Could you check a few things on this model? Use its own coordinates, in mm. Give positions to 0.01 mm unless a question says otherwise; leave off trailing zeros. Loops run counter-clockwise (first coordinate to the right, second up) from the corner with the lowest first, then second, coordinate; pieces in that order, holes last.
1. Imagine slicing it at D-D (y = 12.5). List the corners of the cut face in (x, z) for me.
2. Imagine slicing it at C-C (x = 8). List the corners of the cut face in (y, z) for me, plus the area to 3 significant figures.
3. I need wall thicknesses on line 1 along Y through (x, z) = (13.5, 0.55); line 2 along Y through (x, z) = (-15.25, 1); line 3 along X through (y, z) = (19, 0.8). Which ranges of each line are inside material? Lowest first, please.
4. Imagine slicing it at A-A (x = 15.25). List the corners of the cut face in (y, z) for me.
5. Imagine slicing it at B-B (y = -28). List the corners of the cut face in (x, z) for me.
```python
from build123d import *

# Parameters (mm, degrees)
SKETCH_1_R      = 1.5
EXTRUDE_1_DEPTH = 2


with BuildPart() as part:
    # 草图1 → 凸台-拉伸1 (new body)
    with BuildSketch(Plane.XY):
        with BuildLine():
            Line((-16, 32), (16, 32))
            ThreePointArc((16, 32), (18.121320344, 31.121320344), (19, 29))
            Line((19, 29), (19, -29))
            ThreePointArc((19, -29), (18.121320344, -31.121320344), (16, -32))
            Line((16, -32), (-16, -32))
            ThreePointArc((-16, -32), (-18.121320344, -31.121320344), (-19, -29))
            Line((-19, -29), (-19, 29))
            ThreePointArc((-19, 29), (-18.121320344, 31.121320344), (-16, 32))
        make_face()
        with Locations((-15.25, 28)):
            Circle(SKETCH_1_R, mode=Mode.SUBTRACT)
        with Locations(Location((15.25, 28, 0), (0, 0, 180))):
            Circle(SKETCH_1_R, mode=Mode.SUBTRACT)
        with Locations((15.25, -28)):
            Circle(SKETCH_1_R, mode=Mode.SUBTRACT)
        with Locations(Location((-15.25, -28, 0), (0, 0, 180))):
            Circle(SKETCH_1_R, mode=Mode.SUBTRACT)
        with BuildLine():
            Line((-9, -25), (9, -25))
            ThreePointArc((9, -25), (11, -27), (9, -29))
            Line((9, -29), (-9, -29))
            ThreePointArc((-9, -29), (-11, -27), (-9, -25))
        make_face(mode=Mode.SUBTRACT)
        with BuildLine():
            Line((-9, 25), (9, 25))
            ThreePointArc((9, 25), (11, 27), (9, 29))
            Line((9, 29), (-9, 29))
            ThreePointArc((-9, 29), (-11, 27), (-9, 25))
        make_face(mode=Mode.SUBTRACT)
        with BuildLine():
            Line((-6.617195014, 3), (-13.5, 3))
            ThreePointArc((-13.5, 3), (-13.853553391, 3.146446609), (-14, 3.5))
            Line((-14, 3.5), (-14, 13.609119823))
            ThreePointArc((-14, 13.609119823), (-13.647224638, 14.086953378), (-13.086700376, 13.890515312))
            Line((-13.086700376, 13.890515312), (-6.20389539, 3.781395489))
            ThreePointArc((-6.20389539, 3.781395489), (-6.175212127, 3.266224193), (-6.617195014, 3))
        make_face(mode=Mode.SUBTRACT)
        with BuildLine():
            Line((14, 3.5), (14, 13.609119823))
            ThreePointArc((14, 13.609119823), (13.647224638, 14.086953378), (13.086700376, 13.890515312))
            Line((13.086700376, 13.890515312), (6.20389539, 3.781395489))
            ThreePointArc((6.20389539, 3.781395489), (6.175212127, 3.266224193), (6.617195014, 3))
            Line((6.617195014, 3), (13.5, 3))
            ThreePointArc((13.5, 3), (13.853553391, 3.146446609), (14, 3.5))
        make_face(mode=Mode.SUBTRACT)
        with BuildLine():
            Line((6.617195014, -3), (13.5, -3))
            ThreePointArc((13.5, -3), (13.853553391, -3.146446609), (14, -3.5))
            Line((14, -3.5), (14, -13.609119823))
            ThreePointArc((14, -13.609119823), (13.647224638, -14.086953378), (13.086700376, -13.890515312))
            Line((13.086700376, -13.890515312), (6.20389539, -3.781395489))
            ThreePointArc((6.20389539, -3.781395489), (6.175212127, -3.266224193), (6.617195014, -3))
        make_face(mode=Mode.SUBTRACT)
        with BuildLine():
            Line((-14, -3.5), (-14, -13.609119823))
            ThreePointArc((-14, -13.609119823), (-13.647224638, -14.086953378), (-13.086700376, -13.890515312))
            Line((-13.086700376, -13.890515312), (-6.20389539, -3.781395489))
            ThreePointArc((-6.20389539, -3.781395489), (-6.175212127, -3.266224193), (-6.617195014, -3))
            Line((-6.617195014, -3), (-13.5, -3))
            ThreePointArc((-13.5, -3), (-13.853553391, -3.146446609), (-14, -3.5))
        make_face(mode=Mode.SUBTRACT)
        with BuildLine():
            Line((-8.701953922, 19.5), (-2.5, 19.5))
            ThreePointArc((-2.5, 19.5), (-2.146446609, 19.353553391), (-2, 19))
            Line((-2, 19), (-2, 9.890880177))
            ThreePointArc((-2, 9.890880177), (-2.352775362, 9.413046622), (-2.913299624, 9.609484688))
            Line((-2.913299624, 9.609484688), (-9.115253546, 18.718604511))
            ThreePointArc((-9.115253546, 18.718604511), (-9.143936809, 19.233775807), (-8.701953922, 19.5))
        make_face(mode=Mode.SUBTRACT)
        with BuildLine():
            Line((2, 19), (2, 9.890880177))
            ThreePointArc((2, 9.890880177), (2.352775362, 9.413046622), (2.913299624, 9.609484688))
            Line((2.913299624, 9.609484688), (9.115253546, 18.718604511))
            ThreePointArc((9.115253546, 18.718604511), (9.143936809, 19.233775807), (8.701953922, 19.5))
            Line((8.701953922, 19.5), (2.5, 19.5))
            ThreePointArc((2.5, 19.5), (2.146446609, 19.353553391), (2, 19))
        make_face(mode=Mode.SUBTRACT)
        with BuildLine():
            Line((8.701953922, -19.5), (2.5, -19.5))
            ThreePointArc((2.5, -19.5), (2.146446609, -19.353553391), (2, -19))
            Line((2, -19), (2, -9.890880177))
            ThreePointArc((2, -9.890880177), (2.352775362, -9.413046622), (2.913299624, -9.609484688))
            Line((2.913299624, -9.609484688), (9.115253546, -18.718604511))
            ThreePointArc((9.115253546, -18.718604511), (9.143936809, -19.233775807), (8.701953922, -19.5))
        make_face(mode=Mode.SUBTRACT)
        with BuildLine():
            Line((-2, -19), (-2, -9.890880177))
            ThreePointArc((-2, -9.890880177), (-2.352775362, -9.413046622), (-2.913299624, -9.609484688))
            Line((-2.913299624, -9.609484688), (-9.115253546, -18.718604511))
            ThreePointArc((-9.115253546, -18.718604511), (-9.143936809, -19.233775807), (-8.701953922, -19.5))
            Line((-8.701953922, -19.5), (-2.5, -19.5))
            ThreePointArc((-2.5, -19.5), (-2.146446609, -19.353553391), (-2, -19))
        make_face(mode=Mode.SUBTRACT)
    extrude(amount=EXTRUDE_1_DEPTH)


solid = part.part
```
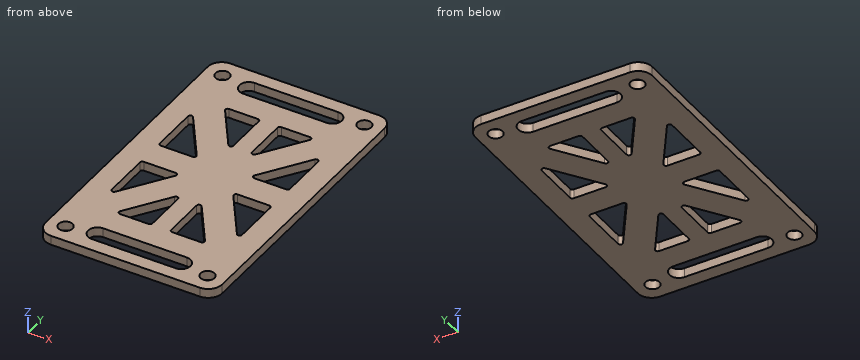
Derived:
1. outline: (-19, 0) - (-14, 0) - (-14, 2) - (-19, 2) - close; (-12.14, 0) - (-4.88, 0) - (-4.88, 2) - (-12.14, 2) - close; (-2, 0) - (2, 0) - (2, 2) - (-2, 2) - close; (4.88, 0) - (12.14, 0) - (12.14, 2) - (4.88, 2) - close; (14, 0) - (19, 0) - (19, 2) - (14, 2) - close
2. outline: (-32, 0) - (-29, 0) - (-29, 2) - (-32, 2) - close; (-25, 0) - (-19.5, 0) - (-19.5, 2) - (-25, 2) - close; (-17.08, 0) - (-6.42, 0) - (-6.42, 2) - (-17.08, 2) - close; (-3, 0) - (3, 0) - (3, 2) - (-3, 2) - close; (6.42, 0) - (17.08, 0) - (17.08, 2) - (6.42, 2) - close; (19.5, 0) - (25, 0) - (25, 2) - (19.5, 2) - close; (29, 0) - (32, 0) - (32, 2) - (29, 2) - close
2. area: 88.6 mm2
3. line 1: y = -32 to -14.11, -3 to 3, 14.11 to 32
3. line 2: y = -32 to -29.5, -26.5 to 26.5, 29.5 to 32
3. line 3: x = -19 to -9.2, -2 to 2, 9.2 to 19
4. outline: (-32, 0) - (-29.5, 0) - (-29.5, 2) - (-32, 2) - close; (-26.5, 0) - (26.5, 0) - (26.5, 2) - (-26.5, 2) - close; (29.5, 0) - (32, 0) - (32, 2) - (29.5, 2) - close
5. outline: (-19, 0) - (-16.75, 0) - (-16.75, 2) - (-19, 2) - close; (-13.75, 0) - (-10.73, 0) - (-10.73, 2) - (-13.75, 2) - close; (10.73, 0) - (13.75, 0) - (13.75, 2) - (10.73, 2) - close; (16.75, 0) - (19, 0) - (19, 2) - (16.75, 2) - close
